Work out the finished part from the listing and answer in its coordinate system (mm). Face numbers are marked on the shaded views. Give positions to 0.01 mm unless a question says otherwise; leave off trailing zeros. Order: outer loops, then holes, each group sorted by start corner. A loop starts at its lowest first (then second) coordinate and runs counter-clockwise, first axis right, second up. Notation, with made-up numbers: (58.25, -38.5) -> (109.25, -38.5) arc R28 cw to (109.25, -11.5) -> close; hole circle Ø2 at (85, 54.5). An arc over 180 degrees is marked (long way). Answer as CSV lines item,"result". Start each with the question number.
1. Find the intervals of material crossed by L1, parallel to Z at x = -9.75, y = -4; L2, parallel to X at y = -4, z = 3.5; L3, parallel to Z at x = 11.7, y = 0, in increasing order.
2. A cutting plane is placed at D-D (z = 8.5). Give the vertices of the cut face in (x, y), then the cut area to 3 significant figures.
3. A cutting plane is placed at C-C (y = 0). Give the vertices of the cut face in (x, z), then the cut area to 3 significant figures.
4. A cutting plane is placed at A-A (x = -1.75). Give the vertices of the cut face in (y, z).
5. A cutting plane is placed at B-B (y = 3.25). Give the vertices of the cut face in (x, z).
6. For a pull along X with two mould halves and no side action, classify the marked faces 1, 2, 3 and 4 as released by +X, released by -X, zero draft, split by the parting line, or undercut.
7. Flat-ended cylindrical pins translate along their axes: pin 1 (10 mm diameter, centred on x = -9, y = -7.5, fed in from +Z); pin 2 (5 mm diameter, centred on y = 0, z = 20, fed in from -X); pin 3 (0.5 mm diameter, centred on y = 0, z = -0.5, fed in from +X); pin 4 (0.8 mm diameter, centred on x = 12, z = 14, fed in from +Y). Find the tip coordinate at first contact, or state that the pin passes through.
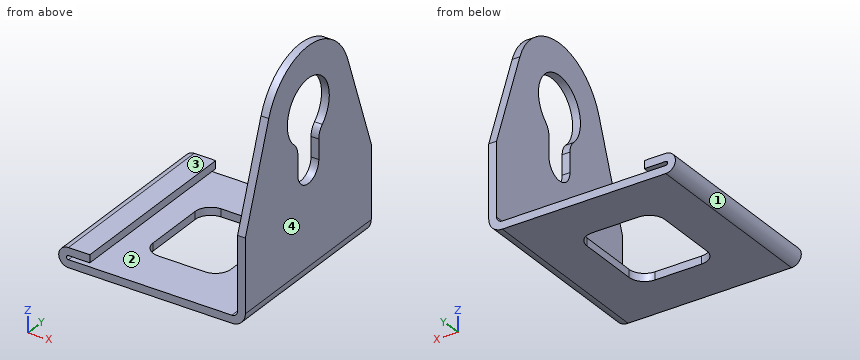
from build123d import *

# Parameters (mm, degrees)
SKETCH1_W               = 21
SKETCH1_H               = 24
BASE_FLANGE1_DEPTH      = 1
EDGE_FLANGE1_DEPTH      = 24
EDGE_FLANGE1_START      = 1
EDGE_FLANGE1_FLAT_DEPTH = 1
HEM1_START              = -12
HEM1_DEPTH              = 24


# Read off the part's stored shape, not the designer's step: Hem1
# Sheet-metal steps are written as plain solids
with BuildPart() as part:
    # Sketch1 → Base-Flange1 (new body)
    with BuildSketch(Plane.XY):
        Rectangle(SKETCH1_W, SKETCH1_H)
        with BuildLine():
            Line((-3, 6), (3, 6))
            ThreePointArc((3, 6), (4.414213562, 5.414213562), (5, 4))
            Line((5, 4), (5, -4))
            ThreePointArc((5, -4), (4.414213562, -5.414213562), (3, -6))
            Line((3, -6), (-3, -6))
            ThreePointArc((-3, -6), (-4.414213562, -5.414213562), (-5, -4))
            Line((-5, -4), (-5, 4))
            ThreePointArc((-5, 4), (-4.414213562, 5.414213562), (-3, 6))
        make_face(mode=Mode.SUBTRACT)
    extrude(amount=-BASE_FLANGE1_DEPTH)

    # Edge-Flange1 bend section (across the edge) → Edge-Flange1 (add)
    with BuildSketch(Plane(origin=(11.2366, -12, 0), x_dir=(-1, 0, 0), z_dir=(0, 1, 0))):
        with BuildLine():
            Line((-1, 0.7366), (0, 0.7366))
            ThreePointArc((0, 0.7366), (0.215745145, 0.215745145), (0.7366, 0))
            Line((0.7366, 0), (0.7366, -1))
            ThreePointArc((0.7366, -1), (-0.491361636, -0.491361636), (-1, 0.7366))
        make_face()
    extrude(amount=EDGE_FLANGE1_DEPTH)

    # Edge-Flange1 profile (on flange) → Edge-Flange1 flat (add)
    with BuildSketch(Plane.YZ.offset(11.2366).offset(EDGE_FLANGE1_START)):
        with BuildLine():
            ThreePointArc((7.540895956, 22.671121147), (0, 28), (-7.540895956, 22.671121147))
            Line((-7.540895956, 22.671121147), (-12, 10.082534632))
            Line((-12, 10.082534632), (-12, 0.7366))
            Line((-12, 0.7366), (12, 0.7366))
            Line((12, 0.7366), (12, 10.082534632))
            Line((12, 10.082534632), (7.540895956, 22.671121147))
        make_face()
        with BuildLine():
            ThreePointArc((2, 13), (0, 11), (-2, 13))
            Line((-2, 13), (-2, 15.527864045))
            ThreePointArc((-2, 15.527864045), (-2.174258142, 16.344360626), (-2.666666667, 17.01857603))
            ThreePointArc((-2.666666667, 17.01857603), (0, 24), (2.666666667, 17.01857603))
            ThreePointArc((2.666666667, 17.01857603), (2.174258142, 16.344360626), (2, 15.527864045))
            Line((2, 15.527864045), (2, 13))
        make_face(mode=Mode.SUBTRACT)
    extrude(amount=-EDGE_FLANGE1_FLAT_DEPTH)

    # Hem1 outline → Hem1 (add)
    with BuildSketch(Plane(origin=(0, 0, 0), x_dir=(1, 0, 0), z_dir=(0, 1, 0)).offset(HEM1_START)):
        with BuildLine():
            Line((-7.75, -1.5), (-7.75, -0.5))
            Line((-7.75, -0.5), (-10.5, -0.5))
            ThreePointArc((-10.5, -0.5), (-10.75, -0.25), (-10.5, 0))
            Line((-10.5, 0), (-10.5, 1))
            ThreePointArc((-10.5, 1), (-11.75, -0.25), (-10.5, -1.5))
            Line((-10.5, -1.5), (-7.75, -1.5))
        make_face()
    extrude(amount=HEM1_DEPTH)


solid = part.part
Answer sheet:
1,L1,"z = -1 to 0, 0.5 to 1.5"
1,L2,"x = 11.24 to 12.24"
1,L3,"z = -0.52 to 11, 24 to 28"
2,outline,"(11.24, -12) -> (12.24, -12) -> (12.24, 12) -> (11.24, 12) -> close"
2,area,"24.0 mm^2"
3,outline,"(-10.5, -1) -> (-5, -1) -> (-5, 0) -> (-10.5, 0) arc R0.25 cw to (-10.5, 0.5) -> (-7.75, 0.5) -> (-7.75, 1.5) -> (-10.5, 1.5) arc R1.25 ccw to start; (5, -1) -> (10.5, -1) arc R1.74 ccw to (12.24, 0.74) -> (12.24, 11) -> (11.24, 11) -> (11.24, 0.74) arc R0.74 cw to (10.5, 0) -> (5, 0) -> close; (11.24, 24) -> (12.24, 24) -> (12.24, 28) -> (11.24, 28) -> close"
3,area,"32.3 mm^2"
4,outline,"(-12, -1) -> (-6, -1) -> (-6, 0) -> (-12, 0) -> close; (6, -1) -> (12, -1) -> (12, 0) -> (6, 0) -> close"
5,outline,"(-10.5, -1) -> (-5, -1) -> (-5, 0) -> (-10.5, 0) arc R0.25 cw to (-10.5, 0.5) -> (-7.75, 0.5) -> (-7.75, 1.5) -> (-10.5, 1.5) arc R1.25 ccw to start; (5, -1) -> (10.5, -1) arc R1.74 ccw to (12.24, 0.74) -> (12.24, 17.67) -> (11.24, 17.67) -> (11.24, 0.74) arc R0.74 cw to (10.5, 0) -> (5, 0) -> close; (11.24, 22.33) -> (12.24, 22.33) -> (12.24, 27.31) -> (11.24, 27.31) -> close"
6,face 1,"released by -X"
6,face 2,"undercut"
6,face 3,"zero draft"
6,face 4,"released by +X"
7,pin 1,"stops at z = 1.5"
7,pin 2,"passes through"
7,pin 3,"stops at x = 11.93"
7,pin 4,"stops at y = 10.75"
